Source: CAD feature listing. Evaluate the final solid. Frame: model axes, mm. A direction names the side the tool comes from. Round coordinates to 2 decimals unless told otherwise and drop trailing zeros. Loops run counter-clockwise (first coordinate to the right, second up) from the corner with the lowest first, then second, coordinate; pieces in that order, holes last. Notation, with made-up numbers: (-12, 6) -> (20, 6) arc R7 cw to (20, 11) -> close; hole circle Ø7 at (56.5, 73). An arc over 180 degrees is marked (long way). Return JSON: item names as keys, results as strings. Group by question number.
```python
from build123d import *

# Parameters (mm, degrees)
SKETCH_1_R          = 44.5
EXTRUDE_1_DEPTH     = 39.2
EXTRUDE_3_DEPTH     = 13.8
SKETCH_4_R          = 2
CUT_EXTRUDE_1_DEPTH = 13.8
SKETCH_5_R          = 2
CUT_EXTRUDE_2_DEPTH = 10
CHAMFER_1_SIZE      = 1
SKETCH_6_R          = 2.5
CUT_EXTRUDE_3_DEPTH = 5
SKETCH_7_W          = 5
SKETCH_7_H          = 20
CUT_EXTRUDE_4_DEPTH = 3
SKETCH_8_R          = 8.75
CUT_EXTRUDE_5_DEPTH = 17


with BuildPart() as part:
    # 草图1 → 凸台-拉伸1 (new body)
    with BuildSketch(Plane(origin=(0, 0, 0), x_dir=(0, 0, -1), z_dir=(1, 0, 0))):
        Circle(SKETCH_1_R)
    extrude(amount=EXTRUDE_1_DEPTH)

    # 草图2 → 凸台-拉伸3 (add)
    with BuildSketch(Plane(origin=(39.2, 0, 0), x_dir=(0, 0, -1), z_dir=(1, 0, 0))):
        with BuildLine():
            Line((-30, 17.036725037), (-30, -17.036725037))
            ThreePointArc((-30, -17.036725037), (34.5, 0), (-30, 17.036725037))
        make_face()
    extrude(amount=EXTRUDE_3_DEPTH)

    # 草图4 → 切除-拉伸1 (cut)
    with BuildSketch(Plane(origin=(39.2, 0, 0), x_dir=(0, 0, -1), z_dir=(1, 0, 0))):
        with Locations((0.484323727, 39.997067774)):
            Circle(SKETCH_4_R)
        with Locations((34.880638633, 19.579097236)):
            Circle(SKETCH_4_R)
        with Locations((34.396314906, -20.417970538)):
            Circle(SKETCH_4_R)
        with Locations((-0.484323727, -39.997067774)):
            Circle(SKETCH_4_R)
        with Locations((-34.880638633, -19.579097236)):
            Circle(SKETCH_4_R)
        with Locations((-34.396314906, 20.417970538)):
            Circle(SKETCH_4_R)
    extrude(amount=-CUT_EXTRUDE_1_DEPTH, mode=Mode.SUBTRACT)

    # 草图5 → 切除-拉伸2 (cut)
    with BuildSketch(Plane(origin=(53, 0, 0), x_dir=(0, 0, -1), z_dir=(1, 0, 0))):
        with Locations((-15, 15)):
            Circle(SKETCH_5_R)
        with Locations((15, 15)):
            Circle(SKETCH_5_R)
        with Locations((15, -15)):
            Circle(SKETCH_5_R)
        with Locations((-15, -15)):
            Circle(SKETCH_5_R)
    extrude(amount=-CUT_EXTRUDE_2_DEPTH, mode=Mode.SUBTRACT)

    # 倒角1
    chamfer_1_edges = [part.edges().sort_by_distance(p)[0] for p in [
        (0, 0, 44.5),
        (39.2, 0, 44.5),
    ]]
    chamfer(chamfer_1_edges, length=CHAMFER_1_SIZE)

    # 草图6 → 切除-拉伸3 (cut)
    with BuildSketch(Plane.ZY):
        with Locations((0, 22)):
            Circle(SKETCH_6_R)
        with Locations((-12.374368671, 12.374368671)):
            Circle(SKETCH_6_R)
        with Locations((22, 0)):
            Circle(SKETCH_6_R)
        with Locations((12.374368671, 12.374368671)):
            Circle(SKETCH_6_R)
        with Locations((0, -22)):
            Circle(SKETCH_6_R)
        with Locations((12.374368671, -12.374368671)):
            Circle(SKETCH_6_R)
        with Locations((-22, 0)):
            Circle(SKETCH_6_R)
        with Locations((-12.374368671, -12.374368671)):
            Circle(SKETCH_6_R)
    extrude(amount=-CUT_EXTRUDE_3_DEPTH, mode=Mode.SUBTRACT)

    # 草图7 → 切除-拉伸4 (cut)
    with BuildSketch(Plane.XY.offset(30)):
        with Locations((44.7, -1.036725037)):
            Rectangle(SKETCH_7_W, SKETCH_7_H)
    extrude(amount=-CUT_EXTRUDE_4_DEPTH, mode=Mode.SUBTRACT)

    # 草图8 → 切除-拉伸5 (cut)
    with BuildSketch(Plane.ZY):
        Circle(SKETCH_8_R)
    extrude(amount=-CUT_EXTRUDE_5_DEPTH, mode=Mode.SUBTRACT)


solid = part.part
```
(1) Pin query (flat end, axial travel): pin 1 (1.5 mm diameter, centred on x = 46, z = -2, fed in from +Y); pin 2 (12 mm diameter, centred on y = -34, z = -23.5, fed in from +X); pin 3 (1 mm diameter, centred on x = 39.5, y = 16.5, fed in from +Z). Return the tip coordinate at first contact, or that it passes through.
(2) Cut plane B-B (x = 35.5). Return loops of the section in (y, z).
(3) Cut plane D-D (x = 7). Return loops of the section in (y, z).
(4) Set-up query: faces 1 (the face through (2.5, 0.1, 19.5)), 2 (the face through (25.4, 20, 34)). Return all of +Z, -Z, +X, -X, +Y, -Y with unobstructed straight access to the full face (end or side cutting, diameter ignored); none if empty.
(5) Mould query, pull axis Y, two halves, no side actions, for faces 3 (the face through (5, 0, 22)), 4 (the face through (19.34, 30.075, 32.798)), 5 (the face through (32.4, 20.18, -36.79)), 6 (the face through (39.2, 0, 32)). Classes: released by +Y, released by -Y, zero draft, split by the parting line, or undercut.
(6) Cut plane A-A (y = 0). Return loops of the section in (x, z), and give its area (3 significant figures).
(7) Ray query, line 1 (Y direction, x = 46.25, z = 15); line 2 (Z direction, x = 49.5, y = 0); line 3 (X direction, y = 10.5, z = 31). Return the intervals inside material, ascending.
Answers follow:
{
 "1": {"pin 1": "y = 34.48", "pin 2": "x = 39.2", "pin 3": "z = 40.5"},
 "2": {"outline": "circle Ø89 at (0, 0); hole circle Ø4 at (-40, 0.48); hole circle Ø4 at (-20.42, -34.4); hole circle Ø4 at (-19.58, 34.88); hole circle Ø4 at (19.58, -34.88); hole circle Ø4 at (20.42, 34.4); hole circle Ø4 at (40, -0.48)"},
 "3": {"outline": "circle Ø89 at (0, 0); hole circle Ø17.5 at (0, 0)"},
 "4": {"face 1": "-X", "face 2": "+X"},
 "5": {"face 3": "undercut", "face 4": "split by the parting line", "face 5": "undercut", "face 6": "zero draft"},
 "6": {"outline": "(0, -43.5) -> (1, -44.5) -> (38.2, -44.5) -> (39.2, -43.5) -> (39.2, -34.5) -> (53, -34.5) -> (53, 30) -> (47.2, 30) -> (47.2, 27) -> (42.2, 27) -> (42.2, 30) -> (39.2, 30) -> (39.2, 43.5) -> (38.2, 44.5) -> (1, 44.5) -> (0, 43.5) -> (0, 24.5) -> (5, 24.5) -> (5, 19.5) -> (0, 19.5) -> (0, 8.75) -> (17, 8.75) -> (17, -8.75) -> (0, -8.75) -> (0, -19.5) -> (5, -19.5) -> (5, -24.5) -> (0, -24.5) -> close", "area": "4,010 mm^2"},
 "7": {"line 1": "-31.07 to -17, -13 to 13, 17 to 31.07", "line 2": "-34.5 to 30", "line 3": "0 to 39.2"}
}
